Design review of the part built by this model. Coordinates are the model's own, in mm. A direction names the side the tool comes from. Round coordinates to 2 decimals unless told otherwise and drop trailing zeros. Write each loop counter-clockwise with the first axis right and the second up, starting at its lowest first coordinate (ties: lowest second). Pieces come first, ordered by that corner, then holes. Notation, with made-up numbers: M 47,50.25 L 97,50.25 A24 cw 97,67.25 Z; hole C 13,13 d4. An arc over 180 degrees is marked long. Use CSV: the item, a comma, the result in double quotes.
from build123d import *

# Parameters (mm, degrees)
Y_KSEKLIK_EKSTR_ZYON1_DEPTH = 24
Y_KSEKLIK_EKSTR_ZYON3_DEPTH = 120
KES_EKSTR_ZYON1_DEPTH       = 120
KES_EKSTR_ZYON2_DEPTH       = 120


with BuildPart() as part:
    # Çizim1 → Yükseklik-Ekstrüzyon1 (new body)
    with BuildSketch(Plane.XY):
        Polygon((18.475208614, 0), (9.237604307, 16), (-9.237604307, 16), (-18.475208614, 0), (-9.237604307, -16), (9.237604307, -16), align=None)
        Polygon((2.309401077, 0), (1.154700538, 2), (-1.154700538, 2), (-2.309401077, 0), (-1.154700538, -2), (1.154700538, -2), align=None, mode=Mode.SUBTRACT)
    extrude(amount=Y_KSEKLIK_EKSTR_ZYON1_DEPTH)

    # Çizim2 → Yükseklik-Ekstrüzyon3 (add)
    with BuildSketch(Plane(origin=(-13.856406461, 8, 0), x_dir=(0, 0, 1), z_dir=(-0.866025404, 0.5, 0))):
        with BuildLine():
            ThreePointArc((20.566689436, 8.632459435), (12.282851611, -2.425053991), (0.070057864, -8.885567992))
            ThreePointArc((0.070057864, -8.885567992), (0, -9.037604307), (0.070057864, -9.189640622))
            ThreePointArc((0.070057864, -9.189640622), (13.640166109, -4.672052834), (23.386017658, 5.795746113))
            ThreePointArc((23.386017658, 5.795746113), (23.418553761, 8.64746431), (20.566689436, 8.632459435))
        make_face()
    extrude(amount=Y_KSEKLIK_EKSTR_ZYON3_DEPTH)

    # Çizim4 → Kes-Ekstrüzyon1 (cut)
    with BuildSketch(Plane.XY.offset(24)):
        with BuildLine():
            Line((-105.114365337, 71.354096261), (-100.895998051, 78.520414233))
            Line((-100.895998051, 78.520414233), (-120.05269231, 81.506783127))
            Line((-120.05269231, 81.506783127), (-133.968493321, 62.353012073))
            Line((-133.968493321, 62.353012073), (-123.727089206, 47.811781803))
            Line((-123.727089206, 47.811781803), (-114.313260633, 55.388064385))
            ThreePointArc((-114.313260633, 55.388064385), (-117.77159569, 68.013605153), (-105.114365337, 71.354096261))
        make_face()
    extrude(amount=-KES_EKSTR_ZYON1_DEPTH, mode=Mode.SUBTRACT)

    # Çizim5 → Kes-Ekstrüzyon2 (cut)
    with BuildSketch(Plane.XY.offset(24)):
        Polygon((9.237604307, 16), (-9.237604307, -16), (-9.237604307, -28.740421499), (42.199790623, -28.740421499), (42.199790623, 12.667995961), align=None)
    extrude(amount=-KES_EKSTR_ZYON2_DEPTH, mode=Mode.SUBTRACT)


solid = part.part
1) For pin 1 Ø5 at (y, z) = (12, 13.5) entering from +X; pin 2 Ø1.2 at (x, z) = (-0.5, 9.5) entering from -Y; pin 3 Ø4 at (x, z) = (-60, 11) entering from +Y, all flat-tipped, find the tip position at first contact; note any pin that passes through.
Answers:
pin 1,"x = 8.37"
pin 2,"y = 2"
pin 3,"y = 32.87"
2) The part is to be moulded in two halves that separate along X. For faces 1 (the face through (-66.24, 35.59, 12.43)), 2 (the face through (-5, 4, 24)), 3 (the face through (-13.92, -7.89, 11.83)), say which applies: released by +X, released by -X, zero draft, split by the parting line, or undercut.
Answers:
face 1,"undercut"
face 2,"zero draft"
face 3,"released by -X"
3) Add section B-B on z = 16.5. Write out the cut boundary in (x, y), then the cut area to 3 significant figures.
Answers:
outline,"M -118.74,65.58 L -15.14,5.77 L -18.48,0 L -9.24,-16 L -1.15,-2 L -2.31,0 L -1.15,2 L 1.15,2 L 9.24,16 L -9.24,16 L -12.88,9.69 L -116.63,69.59 A9.21 ccw Z"
area,"979 mm²"
4) Wall thickness on line 1 along X through (y, z) = (29.5, 1.25); line 2 along Y through (x, z) = (-63, 4.25); line 3 along X through (y, z) = (47, 8.75): over which ranges is each line inside the solid? List them lowest first. Write a range as [from, to].
Answers:
line 1,"[-69.26, -68.17]"
line 2,"[26.46, 27.8]"
line 3,"[-95.79, -91.49]"
5) Machinability: for faces 4 (the face through (-16.168, 3.997, 17.277)), 5 (the face through (-12.7, 10, 8.4)), 6 (the face through (0, 16, 12)), which of the approach directions +Z, -Z, +X, -X, +Y, -Y give a long, thin tool a straight path to every point of the face, cutting with its end or side? Answer none if there is none.
Answers:
face 4,"+Z, -X"
face 5,"-Z, +Y"
face 6,"+Z, -Z, +X, +Y"
6) Add section A-A on z = 7. Write out the cut boundary in (x, y).
Answers:
outline,"M -118.82,61.58 A9.21 ccw -117.89,59.02 L -17.77,1.22 L -18.48,0 L -9.24,-16 L -1.15,-2 L -2.31,0 L -1.15,2 L 1.15,2 L 9.24,16 L -9.24,16 L -16.9,2.73 Z"
